from build123d import *

# Parameters (mm, degrees)
CROQUIS1_R              = 45
SALIENTE_EXTRUIR1_DEPTH = 58
CROQUIS2_R              = 22
SALIENTE_EXTRUIR2_DEPTH = 18.5
SALIENTE_EXTRUIR3_DEPTH = 10.3
CROQUIS4_R              = 2.5
CORTAR_EXTRUIR1_DEPTH   = 115.269878576
CROQUIS5_R              = 3
CORTAR_EXTRUIR2_DEPTH   = 10


with BuildPart() as part:
    # Croquis1 → Saliente-Extruir1 (new body)
    with BuildSketch(Plane.XY):
        with Locations(Location((0, 0, 0), (0, 0, 180))):
            Circle(CROQUIS1_R)
    extrude(amount=SALIENTE_EXTRUIR1_DEPTH)

    # Croquis2 → Saliente-Extruir2 (add)
    with BuildSketch(Plane.XY.offset(58)):
        Circle(CROQUIS2_R)
    extrude(amount=SALIENTE_EXTRUIR2_DEPTH)

    # Croquis3 → Saliente-Extruir3 (add)
    with BuildSketch(Plane.XY.offset(76.5)):
        Polygon((12.701705922, 0), (6.350852961, 11), (-6.350852961, 11), (-12.701705922, 0), (-6.350852961, -11), (6.350852961, -11), align=None)
    extrude(amount=SALIENTE_EXTRUIR3_DEPTH)

    # Croquis4 → Cortar-Extruir1 (cut, through all)
    with BuildSketch(Plane(origin=(9.526279442, 5.5, 0), x_dir=(0, 0, -1), z_dir=(0.8660254037844384, 0.5000000000000003, 0))):
        with Locations(Location((-80.8, 0, 0), (0, 0, 90))):
            Circle(CROQUIS4_R)
    extrude(amount=-CORTAR_EXTRUIR1_DEPTH, mode=Mode.SUBTRACT)

    # Croquis5 → Cortar-Extruir2 (cut)
    with BuildSketch(Plane.XY.offset(58)):
        with Locations((-35.5, 0)):
            Circle(CROQUIS5_R)
        with Locations((35.5, 0)):
            Circle(CROQUIS5_R)
        with Locations((0, 35.5)):
            Circle(CROQUIS5_R)
    extrude(amount=-CORTAR_EXTRUIR2_DEPTH, mode=Mode.SUBTRACT)


solid = part.part
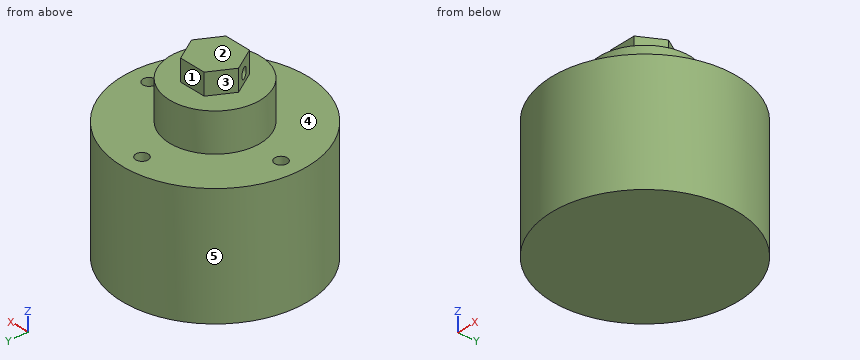
The listing builds one solid part. Answer for the finished solid, in the listing's coordinates (mm). Face numbers are marked on the shaded views. A direction names the side the tool comes from. Coordinates: 2 decimals unless noted, no trailing zeros. Loops run counter-clockwise (first coordinate to the right, second up) from the corner with the lowest first, then second, coordinate; pieces in that order, holes last.
1) Find the intervals of material crossed by L1, parallel to Y at x = 0, z = 54; L2, parallel to Z at x = -16.5, y = -12.5; L3, parallel to Z at x = 16, y = 40, in increasing order.
2) Find section B-B on x = 36.5. Write down the section's boundary in (y, z), then the cut area to 3 significant figures.
3) Find section C-C on z = 22. Write down the section's boundary in (x, y), then the cut area to 3 significant figures.
4) Find section A-A on y = 13. Write down the section's boundary in (x, z).
5) A tool of negligible diameter and unlimited length cuts with its end or side. For the marked faces 1, 2, 3, 4 and 5, from which of +Z, -Z, +X, -X, +Y, -Y can it reach the whole face along a straight path? Write none if from no direction.
6) Flat-ended cylindrical pins translate along their axes: pin 1 Ø5.5 at (x, y) = (35.5, 0) entering from +Z; pin 2 Ø4 at (y, z) = (-14.5, 26.5) entering from +X; pin 3 Ø6.5 at (x, y) = (-34.5, 1) entering from +Z. Find the tip coordinate at first contact, or state that the pin passes through.
7) Find section D-D on y = 23.5. Write down the section's boundary in (x, z), then the cut area to 3 significant figures.
Values:
1. L1: y = -45 to 32.5, 38.5 to 45
1. L2: z = 0 to 76.5
1. L3: z = 0 to 58
2. outline: (-26.32, 0) - (26.32, 0) - (26.32, 58) - (2.83, 58) - (2.83, 48) - (-2.83, 48) - (-2.83, 58) - (-26.32, 58) - close
2. area: 3,000 mm2
3. outline: circle Ø90 at (0, 0)
3. area: 6,360 mm2
4. outline: (-43.08, 0) - (43.08, 0) - (43.08, 58) - (17.75, 58) - (17.75, 76.5) - (-17.75, 76.5) - (-17.75, 58) - (-43.08, 58) - close
5. face 1: +Z, +X, -X, +Y
5. face 2: +Z, +X, -X, +Y, -Y
5. face 3: +Z, -X, +Y
5. face 4: +Z
5. face 5: +Z, -Z
6. pin 1: stops at z = 48
6. pin 2: stops at x = 43.23
6. pin 3: stops at z = 58
7. outline: (-38.38, 0) - (38.38, 0) - (38.38, 58) - (-38.38, 58) - close
7. area: 4,450 mm2
